CAD build for the part. Positions are in the model's coordinates, mm. Round coordinates to 2 decimals unless told otherwise and drop trailing zeros. Write each loop counter-clockwise with the first axis right and the second up, starting at its lowest first coordinate (ties: lowest second). Pieces come first, ordered by that corner, then holes. Notation, with made-up numbers: (70, 49) -> (80, 49) arc R25 ccw to (80, 68) -> close; hole circle Ø10 at (79.5, 37). An arc over 180 degrees is marked (long way). Put each result on its own line as item: value. Start each with the question number.
1. Flat gauge pins, fed straight in: P1, Ø3.5, axis at x = -15.99, z = -11.1, coming from the +Y side; P2, Ø3, axis at y = 10, z = 6, coming from the +X side. Where does each tip first touch, or does it go through?
2. Saw through at D-D on y = 4.25. List the corners of the cut face in (x, z), and give its area (3 significant figures).
3. Saw through at A-A on x = 6.28. List the corners of the cut face in (y, z).
4. Saw through at B-B on y = 17.5. List the corners of the cut face in (x, z), and give its area (3 significant figures).
5. Pull direction Z, two halves, no side cores. Call faces 1 (the flat face through (0, 1, -12.5)), 2 (the cylindrical face through (-7.7, 0.98, -0.07)), 3 (the flat face through (13, 1, 12.5)), 4 (the flat face through (-24.2, 13, 3)): pulls with the +Z half, pulls with the -Z half, needs draft (parallel to the pull), parting line crosses it, or undercut.
6. Drill centre lines: line 1 (Z direction, x = 6.28, y = 1.35); line 2 (Y direction, x = -8.5, z = 0.75); line 3 (X direction, y = 5, z = 3.25). Where is each one in solid material? Low to high. Write a range as from..to.
7. Saw through at C-C on z = 7.25. List the corners of the cut face in (x, y).
from build123d import *

# Parameters (mm, degrees)
SKETCH1_R           = 1.5
BOSS_EXTRUDE1_DEPTH = 1.98
SKETCH2_W           = 1.98
SKETCH2_H           = 25
BOSS_EXTRUDE2_DEPTH = 14.5
SKETCH3_R           = 12.5
BOSS_EXTRUDE5_DEPTH = 1.98
SKETCH4_R           = 3.75
CUT_EXTRUDE1_DEPTH  = 14.5


with BuildPart() as part:
    # Sketch1 → Boss-Extrude1 (new body)
    with BuildSketch(Plane(origin=(0, 0, 0), x_dir=(1, 0, 0), z_dir=(0, 1, 0))):
        with BuildLine():
            Line((16.298685972, -12.5), (26.18, -12.5))
            Line((26.18, -12.5), (26.18, 12.5))
            Line((26.18, 12.5), (16.298685972, 12.5))
            ThreePointArc((16.298685972, 12.5), (15.760169492, 9.6), (15.221653011, 12.5))
            Line((15.221653011, 12.5), (-15.451314028, 12.5))
            ThreePointArc((-15.451314028, 12.5), (-15.989830508, 9.6), (-16.528346989, 12.5))
            Line((-16.528346989, 12.5), (-26.18, 12.5))
            Line((-26.18, 12.5), (-26.18, -12.5))
            Line((-26.18, -12.5), (-16.528346989, -12.5))
            ThreePointArc((-16.528346989, -12.5), (-16.839014022, -9.863518152), (-14.489830508, -11.1))
            ThreePointArc((-14.489830508, -11.1), (-14.75334866, -11.949183513), (-15.451314028, -12.5))
            Line((-15.451314028, -12.5), (-10.920895266, -12.5))
            ThreePointArc((-10.920895266, -12.5), (-10.315854683, -10.110021252), (-8.289830508, -11.514762712))
            ThreePointArc((-8.289830508, -11.514762712), (-8.385089049, -12.040786886), (-8.658765751, -12.5))
            Line((-8.658765751, -12.5), (-4.640895266, -12.5))
            ThreePointArc((-4.640895266, -12.5), (-4.035854683, -10.110021252), (-2.009830508, -11.514762712))
            ThreePointArc((-2.009830508, -11.514762712), (-2.105089049, -12.040786886), (-2.378765751, -12.5))
            Line((-2.378765751, -12.5), (1.559104734, -12.5))
            ThreePointArc((1.559104734, -12.5), (2.164145317, -10.110021252), (4.190169492, -11.514762712))
            ThreePointArc((4.190169492, -11.514762712), (4.094910951, -12.040786886), (3.821234249, -12.5))
            Line((3.821234249, -12.5), (7.799342787, -12.5))
            ThreePointArc((7.799342787, -12.5), (8.336202009, -10.076431428), (10.390169492, -11.470389831))
            ThreePointArc((10.390169492, -11.470389831), (10.284127894, -12.024357313), (9.980996196, -12.5))
            Line((9.980996196, -12.5), (15.221653011, -12.5))
            ThreePointArc((15.221653011, -12.5), (14.910985978, -9.863518152), (17.260169492, -11.1))
            ThreePointArc((17.260169492, -11.1), (16.99665134, -11.949183513), (16.298685972, -12.5))
        make_face()
        with Locations((-18.6, 0)):
            Circle(SKETCH1_R, mode=Mode.SUBTRACT)
        with Locations((-12.4, 0)):
            Circle(SKETCH1_R, mode=Mode.SUBTRACT)
        with Locations((-6.2, 0)):
            Circle(SKETCH1_R, mode=Mode.SUBTRACT)
        with Locations((0.08, 0)):
            Circle(SKETCH1_R, mode=Mode.SUBTRACT)
        with Locations((6.28, 0)):
            Circle(SKETCH1_R, mode=Mode.SUBTRACT)
        with Locations((12.48, -0.044372881)):
            Circle(SKETCH1_R, mode=Mode.SUBTRACT)
        with Locations((18.68, 0)):
            Circle(SKETCH1_R, mode=Mode.SUBTRACT)
    extrude(amount=BOSS_EXTRUDE1_DEPTH)

    # Sketch2 → Boss-Extrude2 (add)
    with BuildSketch(Plane(origin=(0, 1.98, 0), x_dir=(1, 0, 0), z_dir=(0, 1, 0))):
        with Locations((-25.19, 0)):
            Rectangle(SKETCH2_W, SKETCH2_H)
    extrude(amount=BOSS_EXTRUDE2_DEPTH)

    # Sketch3 → Boss-Extrude5 (add)
    with BuildSketch(Plane.ZY.offset(26.18)):
        with Locations((0, 16.48)):
            Circle(SKETCH3_R)
    extrude(amount=-BOSS_EXTRUDE5_DEPTH)

    # Sketch4 → Cut-Extrude1 (cut)
    with BuildSketch(Plane.ZY.offset(26.18)):
        with Locations((0, 16.48)):
            Circle(SKETCH4_R)
    extrude(amount=-CUT_EXTRUDE1_DEPTH, mode=Mode.SUBTRACT)


solid = part.part
Return value:
1. P1: stops at y = 1.98
1. P2: stops at x = -24.2
2. outline: (-26.18, -12.5) -> (-24.2, -12.5) -> (-24.2, 12.5) -> (-26.18, 12.5) -> close
2. area: 49.5 mm^2
3. outline: (0, -12.5) -> (1.98, -12.5) -> (1.98, -1.5) -> (0, -1.5) -> close; (0, 1.5) -> (1.98, 1.5) -> (1.98, 12.5) -> (0, 12.5) -> close
4. outline: (-26.18, -12.46) -> (-24.2, -12.46) -> (-24.2, -3.61) -> (-26.18, -3.61) -> close; (-26.18, 3.61) -> (-24.2, 3.61) -> (-24.2, 12.46) -> (-26.18, 12.46) -> close
4. area: 35.0 mm^2
5. face 1: pulls with the -Z half
5. face 2: undercut
5. face 3: pulls with the +Z half
5. face 4: needs draft
6. line 1: z = -12.5..-1.5, 1.5..12.5
6. line 2: y = 0..1.98
6. line 3: x = -26.18..-24.2
7. outline: (-26.18, 0) -> (26.18, 0) -> (26.18, 1.98) -> (-24.2, 1.98) -> (-24.2, 26.66) -> (-26.18, 26.66) -> close
